```python
from build123d import *

# Parameters (mm, degrees)
BOSS_EXTRUDE1_DEPTH            = 3.18
F_3_2_3_2_DIAMETER_HOLE1_D     = 3.2
F_3_2_3_2_DIAMETER_HOLE1_DEPTH = 3.18
F_10_0_10_DIAMETER_HOLE1_D     = 10
F_10_0_10_DIAMETER_HOLE1_DEPTH = 3.18


with BuildPart() as part:
    # Sketch1 → Boss-Extrude1 (new body)
    with BuildSketch(Plane(origin=(0, 0, 0), x_dir=(1, 0, 0), z_dir=(0, 1, 0))):
        with BuildLine():
            Line((-16.648706397, -9.505239672), (-16.648706397, 9.505239672))
            ThreePointArc((-16.648706397, 9.505239672), (-19.441368429, 14.783464504), (-15.185935574, 18.972725753))
            Line((-15.185935574, 18.972725753), (9.48849845, 38.527527259))
            ThreePointArc((9.48849845, 38.527527259), (15.561102251, 39.197729336), (18.807607076, 34.022220261))
            Line((18.807607076, 34.022220261), (18.807607076, 2.538606169))
            ThreePointArc((18.807607076, 2.538606169), (18.464212779, -3.047132594), (13.154706871, -4.815619005))
            Line((13.154706871, -4.815619005), (-9.89031278, -15.956694023))
            ThreePointArc((-9.89031278, -15.956694023), (-17.95245166, -17.636708108), (-16.648706397, -9.505239672))
        make_face()
        Polygon((-9.148706397, 7.267686973), (5.884312306, 0), (-9.148706397, -7.267686973), align=None, mode=Mode.SUBTRACT)
        Polygon((-3.543212985, 12.88819957), (6.807607076, 7.884113458), (6.807607076, 21.091355578), align=None, mode=Mode.SUBTRACT)
    extrude(amount=BOSS_EXTRUDE1_DEPTH)

    # Ø3.2 (3.2) Diameter Hole1
    with Locations(Plane(origin=(0, 3.18, 0), x_dir=(-1, 0, 0), z_dir=(0, 1, 0))):
        with Locations((-14.5, 0), (14.5, 14.02), (14.5, -14.02)):
            Hole(F_3_2_3_2_DIAMETER_HOLE1_D / 2, depth=F_3_2_3_2_DIAMETER_HOLE1_DEPTH)

    # Ø10.0 (10) Diameter Hole1
    with Locations(Plane(origin=(0, 0, 0), x_dir=(-1, 0, 0), z_dir=(0, -1, 0))):
        with Locations((-10.338071706, 28.394028492)):
            Hole(F_10_0_10_DIAMETER_HOLE1_D / 2, depth=F_10_0_10_DIAMETER_HOLE1_DEPTH)


solid = part.part
```
The listing builds one solid part. Answer for the finished solid, in the listing's coordinates (mm). A direction names the side the tool comes from. Coordinates: 2 decimals unless noted, no trailing zeros. Write each loop counter-clockwise with the first axis right and the second up, starting at its lowest first coordinate (ties: lowest second). Pieces come first, ordered by that corner, then holes. Notation, with made-up numbers: M 16,19 L 74,19 A17 cw 74,40 Z; hole C 55.25,10.5 d8. An arc over 180 degrees is marked long. Use a Markdown table: item, result. Add a question column.
1. Section D-D (y = 1.6) is taken. Give the vertices of the cut face in (x, z), plus the area to 3 significant figures.
2. Section B-B (z = -14.02) is taken. Give the vertices of the cut face in (x, y).
3. Section A-A (x = 14.5) is taken. Give the vertices of the cut face in (y, z).
4. Section C-C (z = -29) is taken. Give the vertices of the cut face in (x, y), plus the area to 3 significant figures.
5. Which of the six approach directions +Z, -Z, +X, -X, +Y, -Y give full straight-line access (tool end or side, diameter ignored) to faces 1 (the flat face through (-16.649, 2, 0)), 2 (the flat face through (-3.021, 1.568, -28.613)), 3 (the flat face through (-1.527, 1.568, 3.583))?
6. Given P1, Ø9, axis at x = 10.34, z = -28.39, coming from the -Y side; P2, Ø8, axis at x = -15.5, z = 13, coming from the +Y side; P3, Ø1, axis at y = 2, z = 2.5, coming from the +X side, each flat-ended and moving along its own axis, determine where each tip first touches the part or whether it passes through.
7. For a pull along Z with two mould halves and no side action, classify faces 4 (the cylindrical face through (18.5, 1.6, 3)), 5 (the cylindrical face through (15.48, 1.568, -39.236)), 6 (the cylindrical face through (-16.1, 1.6, 14.1)) as +Z half, -Z half, draft (parallel to the pull), parting line (faces both ways), or undercut.
8. Straight lines are drawn through the part: line 1 along Z through (x, y) = (1.5, 2.85) (3 decimals); line 2 along Z through (x, y) = (14.5, 2.05); line 3 along X through (y, z) = (1.1, -2). For each, find the intervals that lie inside material, in ascending order. Write a range as [from, to].
Data:
| question | item | result |
|---|---|---|
| 1 | outline | M -16.65,-9.51 A5 ccw -15.19,-18.97 L 9.49,-38.53 A5.75 ccw 18.81,-34.02 L 18.81,-2.54 A5 ccw 13.15,4.82 L -9.89,15.96 A5 ccw long -16.65,9.51 Z; hole C -14.5,-14.02 d3.2; hole C -14.5,14.02 d3.2; hole M -9.15,-7.27 L 5.88,0 L -9.15,7.27 Z; hole M -3.54,-12.89 L 6.81,-21.09 L 6.81,-7.88 Z; hole C 10.34,-28.39 d10; hole C 14.5,0 d3.2 |
| 1 | area | 1,250 mm2 |
| 2 | outline | M -19.5,0 L -16.1,0 L -16.1,3.18 L -19.5,3.18 Z; M -12.9,0 L -2.12,0 L -2.12,3.18 L -12.9,3.18 Z; M 6.81,0 L 18.81,0 L 18.81,3.18 L 6.81,3.18 Z |
| 3 | outline | M 0,-39.59 L 3.18,-39.59 L 3.18,-31.17 L 0,-31.17 Z; M 0,-25.62 L 3.18,-25.62 L 3.18,-1.6 L 0,-1.6 Z; M 0,1.6 L 3.18,1.6 L 3.18,5 L 0,5 Z |
| 4 | outline | M -2.53,0 L 5.37,0 L 5.37,3.18 L -2.53,3.18 Z; M 15.3,0 L 18.81,0 L 18.81,3.18 L 15.3,3.18 Z |
| 4 | area | 36.3 mm2 |
| 5 | face 1 | -X, +Y, -Y |
| 5 | face 2 | -Z, -X, +Y, -Y |
| 5 | face 3 | +Y, -Y |
| 6 | P1 | passes through |
| 6 | P2 | stops at y = 3.18 |
| 6 | P3 | stops at x = 19.08 |
| 7 | face 4 | parting line |
| 7 | face 5 | -Z half |
| 7 | face 6 | undercut |
| 8 | line 1 | z = [-32.197, -16.885], [-10.45, -2.12], [2.12, 10.45] |
| 8 | line 2 | z = [-39.59, -31.17], [-25.62, -1.6], [1.6, 5] |
| 8 | line 3 | x = [-16.65, -9.15], [1.75, 19.08] |
